For this review, take the finished solid that the model builds, in its own axes (mm). A direction names the side the tool comes from. Coordinates: 2 decimals unless noted, no trailing zeros. Loops run counter-clockwise (first coordinate to the right, second up) from the corner with the lowest first, then second, coordinate; pieces in that order, holes last. Notation, with made-up numbers: (39.25, 75.25) - (96.25, 75.25) arc R19 cw to (96.25, 92.25) - close; hole circle Ø9 at (-7.5, 11.5). An arc over 180 degrees is marked (long way). Use one line per item in the form item = value. Start each with the question number.
1. Machinability: for faces 5 (the face through (1.35, 5.54, -12.72)), 6 (the face through (1.42, 3.94, 2.12)), which of the approach directions +Z, -Z, +X, -X, +Y, -Y give a long, thin tool a straight path to every point of the face, cutting with its end or side? Answer none if there is none.
2. Add section B-B on y = 4.5. Give the boundary of the cut face in (x, z), and give its area (3 significant figures).
3. Draft analysis for pull direction Z (two halves, no side actions). For faces 1 (the face through (-5, 0, 0)), 2 (the face through (-8.618, 2.958, 20.784)), 3 (the face through (-2, 3, -15)), 4 (the face through (14, 3, -3)), state which applies: +Z half, -Z half, draft (parallel to the pull), parting line (faces both ways), or undercut.
4. For pin 1 Ø1 at (y, z) = (5, 5) entering from -X; pin 2 Ø2.5 at (x, z) = (8, 12) entering from +Y; pin 3 Ø1 at (x, y) = (16.5, 5) entering from +Z, all flat-tipped, find the tip position at first contact; note any pin that passes through.
5. Add section A-A on z = 0. Give the boundary of the cut face in (x, y), and give its area (3 significant figures).
6. Add section C-C on z = 13. Count the separate pieces of the cut face and the enclosed holes in it, and give its area (3 significant figures).
7. To check wall thickness, follow probe 1 along X at (y, z) = (2, -6); probe 2 along X at (y, z) = (4.25, -9); probe 3 along X at (y, z) = (1.5, 0). State the ranges of each line that lie inside material, in increasing order.
```python
from build123d import *

# Parameters (mm, degrees)
SKETCH1_R           = 22.5
SKETCH1_R_2         = 2.65
BOSS_EXTRUDE1_DEPTH = 8
SKETCH2_R           = 4.5
CUT_EXTRUDE1_DEPTH  = 5
CHAMFER1_SIZE       = 2
CUT_EXTRUDE3_DEPTH  = 33.810059595


with BuildPart() as part:
    # Sketch1 → Boss-Extrude1 (new body)
    with BuildSketch(Plane(origin=(0, 0, 0), x_dir=(1, 0, 0), z_dir=(0, 1, 0))):
        with Locations(Location((0, 0, 0), (0, 0, 270))):
            Circle(SKETCH1_R)
        with Locations(Location((0, 17.013016167, 0), (0, 0, 270))):
            Circle(SKETCH1_R_2, mode=Mode.SUBTRACT)
        with Locations(Location((-16.180339887, 5.257311121, 0), (0, 0, 270))):
            Circle(SKETCH1_R_2, mode=Mode.SUBTRACT)
        with Locations(Location((-10, -13.763819205, 0), (0, 0, 270))):
            Circle(SKETCH1_R_2, mode=Mode.SUBTRACT)
        with Locations(Location((10, -13.763819205, 0), (0, 0, 270))):
            Circle(SKETCH1_R_2, mode=Mode.SUBTRACT)
        with Locations(Location((16.180339887, 5.257311121, 0), (0, 0, 270))):
            Circle(SKETCH1_R_2, mode=Mode.SUBTRACT)
    extrude(amount=BOSS_EXTRUDE1_DEPTH)

    # Sketch2 → Cut-Extrude1 (cut)
    with BuildSketch(Plane(origin=(0, 8, 0), x_dir=(1, 0, 0), z_dir=(0, 1, 0))):
        with Locations(Location((-16.180339887, 5.257311121, 0), (0, 0, 270))):
            Circle(SKETCH2_R)
        with Locations(Location((0, 17.013016167, 0), (0, 0, 270))):
            Circle(SKETCH2_R)
        with Locations(Location((16.180339887, 5.257311121, 0), (0, 0, 270))):
            Circle(SKETCH2_R)
        with Locations(Location((10, -13.763819205, 0), (0, 0, 270))):
            Circle(SKETCH2_R)
        with Locations(Location((-10, -13.763819205, 0), (0, 0, 270))):
            Circle(SKETCH2_R)
    extrude(amount=-CUT_EXTRUDE1_DEPTH, mode=Mode.SUBTRACT)

    # Chamfer1
    # the kernel refuses this chamfer: 2 mm, written as the material it takes off along each edge
    with BuildSketch(Plane(origin=(0, 8, 0), x_dir=(0, 0, 1), z_dir=(-1, 0, 0))) as chamfer1_piece_1:
        Polygon((22.5, -CHAMFER1_SIZE), (22.5 - CHAMFER1_SIZE, 0), (22.5, 0), align=None)
    revolve(axis=Axis((0, 8, 0), (0, 1, 0)), mode=Mode.SUBTRACT)

    # Sketch3 → Cut-Extrude3 (cut, through all)
    with BuildSketch(Plane.XZ):
        with BuildLine():
            Line((-0.154470077, -2.545317072), (-2.373006508, -0.933456004))
            ThreePointArc((-2.373006508, -0.933456004), (1.498852393, 2.062993336), (-0.154470077, -2.545317072))
        make_face()
    extrude(amount=-CUT_EXTRUDE3_DEPTH, mode=Mode.SUBTRACT)


solid = part.part
```
Conclusion:
q1.face_5 = +Y
q1.face_6 = +Y, -Y
q2.outline = circle Ø45 at (0, 0); hole circle Ø9 at (-16.18, -5.26); hole circle Ø9 at (-10, 13.76); hole circle Ø9 at (0, -17.01); hole (-2.37, -0.93) - (-0.15, -2.55) arc R2.55 ccw (long way) to start; hole circle Ø9 at (10, 13.76); hole circle Ø9 at (16.18, -5.26)
q2.area = 1,250 mm^2
q3.face_1 = draft
q3.face_2 = parting line
q3.face_3 = undercut
q3.face_4 = undercut
q4.pin_1 = -22.05
q4.pin_2 = 3
q4.pin_3 = 15.82
q5.outline = (-22.5, 0) - (-2.55, 0) - (-2.55, 8) - (-20.5, 8) - (-22.5, 6) - close; (2.55, 0) - (22.5, 0) - (22.5, 6) - (20.5, 8) - (2.55, 8) - close
q5.area = 315 mm^2
q6.separate_pieces = 3
q6.enclosed_holes = 0
q6.area = 170 mm^2
q7.probe_1 = -21.69 to -18.72, -13.64 to 13.64, 18.72 to 21.69
q7.probe_2 = -20.62 to -18.68, -13.68 to 13.68, 18.68 to 20.62
q7.probe_3 = -22.5 to -2.55, 2.55 to 22.5
